Input: part model. Units: mm. Frame: model coordinates. A direction names the side the tool comes from. Round coordinates to 2 decimals unless told otherwise and drop trailing zeros. Loops run counter-clockwise (first coordinate to the right, second up) from the corner with the lowest first, then second, coordinate; pieces in that order, holes last. Notation, with made-up numbers: (27.25, 14) -> (78.25, 14) arc R19 cw to (78.25, 46) -> close; hole circle Ø8 at (-27, -19.5). An arc over 180 degrees is marked (long way). One line per question, with ' | ' between items. Start each with the question number.
Q1. Cut plane A-A on z = 5.75. Return loops of the section in (x, y), and give its area (3 significant figures).
Q2. Mould query, pull axis Y, two halves, no side actions, for faces 1 (the face through (0, 10, 5)), 2 (the face through (0, -11, 6)), 3 (the face through (-4.4, -10.5, 2.5)), 4 (the face through (-19.293, -0.149, 2.465)). Classes: pulls with the +Y half, pulls with the -Y half, needs draft (parallel to the pull), parting line crosses it, or undercut.
Q3. Cut plane C-C on x = -5. Return loops of the section in (y, z).
Q4. Material intervals for L1, parallel to Y at x = -9, z = 0.5; L2, parallel to Z at x = -6.5, y = 0; L3, parallel to Y at x = 16.5, z = 0.25, sorted ascending.
Q5. Cut plane D-D on y = -1.25. Return loops of the section in (x, z), and give its area (3 significant figures).
Q6. Cut plane B-B on z = 0.75. Return loops of the section in (x, y) (1 decimal), and give its area (3 significant figures).
Q7. Contact query for flat-ended pins moving along their axis: P1, Ø1, axis at y = 5, z = 6.5, coming from the -X side; P2, Ø0.5, axis at y = 10.5, z = 4, coming from the -X side; P3, Ø12, axis at x = -2.5, y = 1.5, coming from the +Z side; P4, Ø4, axis at y = -6, z = 3, coming from the -X side. Output: stop coordinate, or through.
Q8. Access query for faces 5 (the face through (-0.38, -9.46, 7.54)), 6 (the face through (-20, 0, 5)), 7 (the face through (1.651, 10.5, 5.6)). Directions: +Z, -Z, +X, -X, +Y, -Y. A direction counts if a zero-diameter tool reaches every point of the face in a straight line with its end or side. Return the directions, or none.
Solid Edge part; units mm, degrees
sketch "Sketch1" plane through (0, 0, 0) normal (0, 0, 1) x (1, 0, 0)
  arc A0 (-16.6681, 11) -> (-16.6681, -11) centre (-1.7936, 0) ccw
  line L0 (-16.6681, -11) -> (15.97, -11)
  arc A1 (15.97, -11) -> (15.97, 11) centre (1.0955, 0) ccw
  line L1 (15.97, 11) -> (-16.6681, 11)
extrude "Protrusion1" add sketch "Sketch1" against normal blind 1
sketch "Sketch2" plane through (0, 0, 0) normal (0, 0, 1) x (1, 0, 0)
  arc A0 (-16.155, 10) -> (-16.155, -10) centre (-1.7936, 0) ccw
  line L0 (-16.155, -10) -> (15.4569, -10)
  arc A1 (15.4569, -10) -> (15.4569, 10) centre (1.0955, 0) ccw
  line L1 (15.4569, 10) -> (-16.155, 10)
  arc A2 (-16.6681, 11) -> (-16.6681, -11) centre (-1.7936, 0) ccw
  line L2 (-16.6681, -11) -> (15.97, -11)
  arc A3 (15.97, -11) -> (15.97, 11) centre (1.0955, 0) ccw
  line L3 (15.97, 11) -> (-16.6681, 11)
extrude "ProtrusioneEstrusa_3" add sketch "Sketch2" along normal blind 5
sketch "Sketch3" plane through (-0.3491, -11, 2) normal (0, -1, 0) x (1, 0, 0)
  line L0 (-6.0472, 3) -> (-6.0472, 0.5)
  line L1 (-6.0472, 0.5) -> (6.0472, 0.5)
  line L2 (6.0472, 0.5) -> (6.0472, 3)
  line L3 (6.0472, 3) -> (-6.0472, 3)
extrude "ScavoEstrusione_1" cut sketch "Sketch3" along normal mid plane 65.044
sketch "Sketch4" plane through (-0.3491, -11, 2) normal (0, -1, 0) x (1, 0, 0)
  line L0 (2, 6.75) -> (2, 0.5)
  line L1 (2, 0.5) -> (0, 0.5)
  line L2 (0, 0.5) -> (-2, 0.5)
  line L3 (-2, 0.5) -> (-2, 6.75)
  line L4 (-2, 6.75) -> (0, 6.75)
  line L5 (0, 6.75) -> (2, 6.75)
extrude "Protrusion2" add sketch "Sketch4" against normal up to vertex (1 mm away)
sketch "Sketch5" plane through (-0.3491, 11, 2) normal (0, 1, 0) x (-1, 0, 0)
  line L0 (-2, 6.75) -> (2, 6.75)
  line L1 (2, 6.75) -> (2, 0.5)
  line L2 (2, 0.5) -> (-2, 0.5)
  line L3 (-2, 0.5) -> (-2, 6.75)
extrude "Protrusion3" add sketch "Sketch5" against normal up to vertex (1 mm away)
sketch "Sketch6" plane through (-2.3491, -10.5, 5.625) normal (-1, 0, 0) x (0, 0, 1)
  line L0 (0.8784, 1.5) -> (3.125, 0.5)
  line L1 (3.125, 0.5) -> (0.8784, 0.5)
  line L2 (0.8784, 0.5) -> (0.8784, 1.5)
  line L3 (3.125, 20.5) -> (0.825, 20.5)
  line L4 (0.825, 20.5) -> (0.825, 19.5)
  line L5 (0.825, 19.5) -> (3.125, 20.5)
extrude "Protrusion4" add sketch "Sketch6" against normal up to vertex (4 mm away)
fillet "Rotondo_1" radius 0.5 2 edges at (-0.3491, -10, 8.75) (-0.3491, 10, 8.75)
fillet "Rotondo_2" radius 0.1 2 edges at (-0.3491, -9, 6.5034) (-0.3491, 9, 6.45)
Results:
1) outline: (-2.35, -11) -> (1.65, -11) -> (1.65, -10) -> (-2.35, -10) -> close; (-2.35, 10) -> (1.65, 10) -> (1.65, 11) -> (-2.35, 11) -> close | area: 8.00 mm^2
2) face 1: undercut | face 2: pulls with the -Y half | face 3: needs draft | face 4: undercut
3) outline: (-11, -1) -> (11, -1) -> (11, 2.5) -> (10, 2.5) -> (10, 0) -> (-10, 0) -> (-10, 2.5) -> (-11, 2.5) -> close
4) L1: -11 to -10, 10 to 11 | L2: -1 to 0 | L3: -10.24 to -8.3, 8.3 to 10.24
5) outline: (-20.25, -1) -> (19.55, -1) -> (19.55, 5) -> (18.55, 5) -> (18.55, 0) -> (-19.25, 0) -> (-19.25, 5) -> (-20.25, 5) -> close | area: 49.8 mm^2
6) outline: (-16.7, -11) -> (16, -11) arc R18.5 ccw to (16, 11) -> (-16.7, 11) arc R18.5 ccw to start; hole (-16.2, -10) -> (15.5, -10) arc R17.5 ccw to (15.5, 10) -> (-16.2, 10) arc R17.5 ccw to start | area: 109 mm^2
7) P1: through | P2: x = -17.19 | P3: z = 0 | P4: x = -19.86
8) face 5: +Z, +X, -X | face 6: +Z, -X, +Y, -Y | face 7: +Z, +Y, -Y
